Input: dimensioned drawing with shaded views. Units: mm. Origin: part minimum x, y, z. A direction names the side the tool comes from. Round coordinates to 2 decimals unless told otherwise and drop trailing zeros. Write each loop counter-clockwise with the first axis right and the second up, starting at its lowest first coordinate (ties: lowest second). Pieces come first, ordered by that corner, then holes. Notation, with made-up numbers: M -32.5,12.5 L -20.5,12.5 A34 cw -20.5,47.5 Z; hole C 59,38 d9. An arc over 180 degrees is marked long. Answer in a Markdown table with one row per item. Add a question column.
Item 1: Mould query, pull axis Z, two halves, no side actions, for the marked faces 1, 2 and 3. Classes: released by +Z, released by -Z, zero draft, split by the parting line, or undercut.
Item 2: Set-up query: the marked faces 4, 5 and 6. Return all of +Z, -Z, +X, -X, +Y, -Y with unobstructed straight access to the full face (end or side cutting, diameter ignored); none if empty.
Item 3: Cut plane C-C on y = 27.5. Return loops of the section in (x, z), and give its area (3 significant figures).
Item 4: Cut plane D-D on x = 9.5. Return loops of the section in (y, z).
Item 5: Material intervals for probe 1 along Y at (x, z) = (4.5, 1); probe 2 along Y at (x, z) = (4.5, 3); probe 3 along Z at (x, y) = (9, 9), sorted ascending.
Item 6: Cut plane B-B on z = 7.5. Return loops of the section in (x, y).
Item 7: Contact query for flat-ended pins moving along their axis: pin 1 (4.5 mm diameter, centred on y = 1, z = 8, fed in from +X); pin 2 (3.5 mm diameter, centred on x = 7, y = 37, fed in from -Z); pin 3 (2.5 mm diameter, centred on x = 7, y = 37, fed in from +Z). Output: stop coordinate, or through.
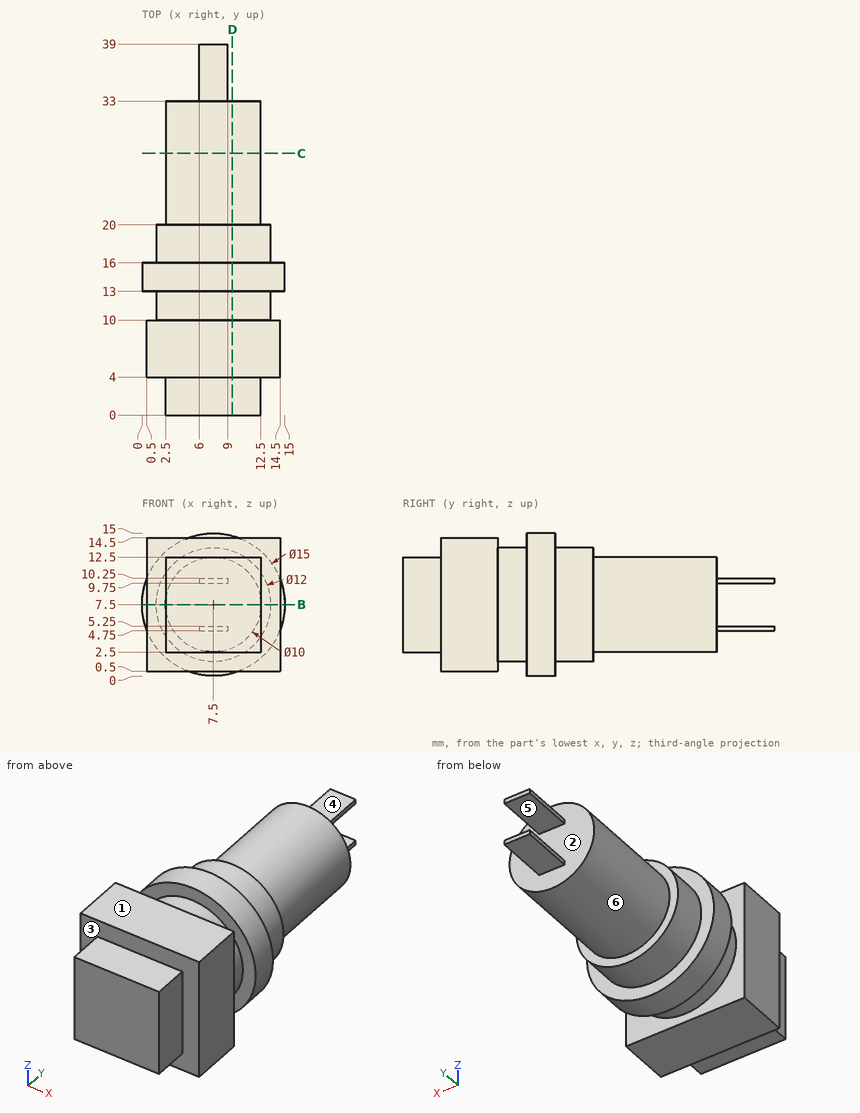
Results below:
| question | item | result |
|---|---|---|
| 1 | face 1 | released by +Z |
| 1 | face 2 | undercut |
| 1 | face 3 | zero draft |
| 2 | face 4 | +Z, +X, -X, +Y |
| 2 | face 5 | +X, -X, +Y |
| 2 | face 6 | +Y |
| 3 | outline | C 7.5,7.5 d10 |
| 3 | area | 78.5 mm2 |
| 4 | outline | M 0,2.5 L 4,2.5 L 4,0.5 L 10,0.5 L 10,1.84 L 13,1.84 L 13,0.27 L 16,0.27 L 16,1.84 L 20,1.84 L 20,2.92 L 33,2.92 L 33,12.08 L 20,12.08 L 20,13.16 L 16,13.16 L 16,14.73 L 13,14.73 L 13,13.16 L 10,13.16 L 10,14.5 L 4,14.5 L 4,12.5 L 0,12.5 Z |
| 5 | probe 1 | 4 to 10, 13 to 16 |
| 5 | probe 2 | 0 to 20 |
| 5 | probe 3 | 0.5 to 14.5 |
| 6 | outline | M 0,13 L 1.5,13 L 1.5,10 L 0.5,10 L 0.5,4 L 2.5,4 L 2.5,0 L 12.5,0 L 12.5,4 L 14.5,4 L 14.5,10 L 13.5,10 L 13.5,13 L 15,13 L 15,16 L 13.5,16 L 13.5,20 L 12.5,20 L 12.5,33 L 2.5,33 L 2.5,20 L 1.5,20 L 1.5,16 L 0,16 Z |
| 7 | pin 1 | x = 12.5 |
| 7 | pin 2 | z = 4.75 |
| 7 | pin 3 | z = 10.25 |
